Source: CAD feature listing. Evaluate the final solid. Frame: model axes, mm. A direction names the side the tool comes from. Coordinates: 2 decimals unless noted, no trailing zeros. Write each loop counter-clockwise with the first axis right and the second up, starting at its lowest first coordinate (ties: lowest second). Pieces come first, ordered by that corner, then holes. Notation, with made-up numbers: (36.25, 81.25) - (67.25, 81.25) arc R33 ccw to (67.25, 114.25) - close; hole circle Ø8 at (62.25, 60.25). An arc over 180 degrees is marked (long way). One line per question, with ' | ' between items. Start each with the question number.
Q1. Line query: line 1 (X direction, y = 41, z = 39); line 2 (Z direction, x = 6.75, y = -15.5); line 3 (Z direction, x = -6, y = -41.5). Output: solid intervals per line, ascending.
Q2. Contact query for flat-ended pins moving along their axis: P1, Ø8, axis at x = 0, y = -40, coming from the -Z side; P2, Ø4, axis at x = 0, y = 0, coming from the +Z side; P3, Ø1, axis at x = -1, y = 36, coming from the +Z side. Output: stop coordinate, or through.
Q3. Access query for faces 1 (the face through (-6, -30, 20)), 2 (the face through (-4.5, 12, 25)), 3 (the face through (-0.54, 37.56, -1.97)). Directions: +Z, -Z, +X, -X, +Y, -Y. A direction counts if a zero-diameter tool reaches every point of the face in a straight line with its end or side. Return the directions, or none.
Q4. Cut plane B-B, the plane z = 24. Return loops of the section in (x, y).
Q5. Cut plane D-D, the plane z = 4.5. Return loops of the section in (x, y), plus the area to 3 significant figures.
Q6. Cut plane A-A, the plane y = 40. Return loops of the section in (x, z).
Q7. Cut plane C-C, the plane y = 7.5. Return loops of the section in (x, z).
Q8. Draft query along Y for faces 4 (the face through (-5, -60, 13)), 5 (the face through (4, 1, -4)), 6 (the face through (-5.7, -39.8, 2.5)), 7 (the face through (-5.73, 57.15, 46.99)). Return one class per face: +Y half, -Y half, draft (parallel to the pull), parting line (faces both ways), or undercut.
```python
from build123d import *

# Parameters (mm, degrees)
SKETCH_1_W          = 14.5
SKETCH_1_H          = 120
SKETCH_1_R          = 2.5
SKETCH_1_W_2        = 2.5
EXTRUDE_1_DEPTH     = 4
SKETCH_1_3_W        = 2.5
SKETCH_1_3_H        = 120
EXTRUDE_2_DEPTH     = 50
FILLET_1_R          = 10
CUT_EXTRUDE_1_DEPTH = 50
CHAMFER_1_SIZE      = 1


with BuildPart() as part:
    # Sketch 1 → Extrude 1 (new body)
    # profile 1 of 2: a face of its own
    with BuildSketch(Plane.XY):
        with Locations((2.75, 0)):
            Rectangle(SKETCH_1_W, SKETCH_1_H)
        with Locations((0, -40)):
            Circle(SKETCH_1_R, mode=Mode.SUBTRACT)
        Circle(SKETCH_1_R, mode=Mode.SUBTRACT)
        with Locations((0, 40)):
            Circle(SKETCH_1_R, mode=Mode.SUBTRACT)
    # profile 2 of 2: a face of its own
    with BuildSketch(Plane.XY):
        with Locations((-5.75, 0)):
            Rectangle(SKETCH_1_W_2, SKETCH_1_H)
    extrude(amount=-EXTRUDE_1_DEPTH)

    # Sketch 1_3 → Extrude 2 (add)
    with BuildSketch(Plane.XY):
        with Locations((-5.75, 0)):
            Rectangle(SKETCH_1_3_W, SKETCH_1_3_H)
    extrude(amount=EXTRUDE_2_DEPTH)

    # Fillet 1
    fillet_1_edges = [part.edges().sort_by_distance(p)[0] for p in [
        (10, 60, -2),
        (10, -60, -2),
        (-5.75, 60, 50),
        (-5.75, -60, 50),
    ]]
    fillet(fillet_1_edges, radius=FILLET_1_R)

    # Sketch 2 → Cut-Extrude 1 (cut)
    with BuildSketch(Plane(origin=(-4.5, 0, 0), x_dir=(0, 0, -1), z_dir=(1, 0, 0))):
        with BuildLine():
            Line((-12.5, -50), (-27.5, -50))
            ThreePointArc((-27.5, -50), (-37.5, -40), (-27.5, -30))
            Line((-27.5, -30), (-12.5, -30))
            ThreePointArc((-12.5, -30), (-2.5, -40), (-12.5, -50))
        make_face()
        with BuildLine():
            Line((-12.5, -10), (-27.5, -10))
            ThreePointArc((-27.5, -10), (-37.5, 0), (-27.5, 10))
            Line((-27.5, 10), (-12.5, 10))
            ThreePointArc((-12.5, 10), (-2.5, 0), (-12.5, -10))
        make_face()
        with BuildLine():
            Line((-12.5, 30), (-27.5, 30))
            ThreePointArc((-27.5, 30), (-37.5, 40), (-27.5, 50))
            Line((-27.5, 50), (-12.5, 50))
            ThreePointArc((-12.5, 50), (-2.5, 40), (-12.5, 30))
        make_face()
    extrude(amount=-CUT_EXTRUDE_1_DEPTH, mode=Mode.SUBTRACT)

    # Chamfer 1
    chamfer_1_edges = [part.edges().sort_by_distance(p)[0] for p in [
        (-7, 0, -4),
    ]]
    chamfer(chamfer_1_edges, length=CHAMFER_1_SIZE)


solid = part.part
```
Reply:
1) line 1: x = -7 to -4.5 | line 2: z = -4 to 0 | line 3: z = -4 to 2.61, 37.39 to 50
2) P1: stops at z = -4 | P2: passes through | P3: stops at z = 0
3) face 1: +X, -X | face 2: +Z, +X, +Y, -Y | face 3: +Z, -Z
4) outline: (-7, -60) - (-4.5, -60) - (-4.5, -50) - (-7, -50) - close; (-7, -30) - (-4.5, -30) - (-4.5, -10) - (-7, -10) - close; (-7, 10) - (-4.5, 10) - (-4.5, 30) - (-7, 30) - close; (-7, 50) - (-4.5, 50) - (-4.5, 60) - (-7, 60) - close
5) outline: (-7, -60) - (-4.5, -60) - (-4.5, -46) - (-7, -46) - close; (-7, -34) - (-4.5, -34) - (-4.5, -6) - (-7, -6) - close; (-7, 6) - (-4.5, 6) - (-4.5, 34) - (-7, 34) - close; (-7, 46) - (-4.5, 46) - (-4.5, 60) - (-7, 60) - close | area: 210 mm^2
6) outline: (-7, -3) - (-6, -4) - (-2.5, -4) - (-2.5, 0) - (-4.5, 0) - (-4.5, 2.5) - (-7, 2.5) - close; (-7, 37.5) - (-4.5, 37.5) - (-4.5, 50) - (-7, 50) - close; (2.5, -4) - (10, -4) - (10, 0) - (2.5, 0) - close
7) outline: (-7, -3) - (-6, -4) - (10, -4) - (10, 0) - (-4.5, 0) - (-4.5, 5.89) - (-7, 5.89) - close; (-7, 34.11) - (-4.5, 34.11) - (-4.5, 50) - (-7, 50) - close
8) face 4: -Y half | face 5: draft | face 6: undercut | face 7: +Y half
